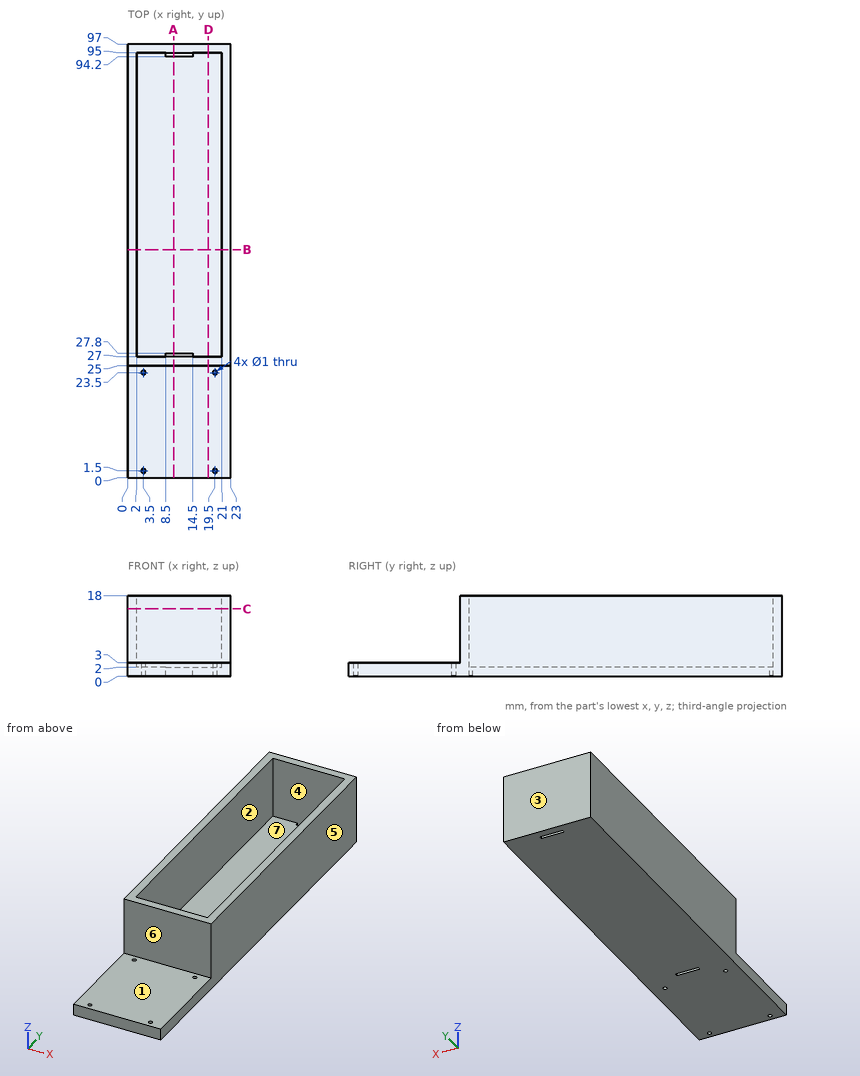
Geometry: see drawing. Coordinates: mm, zero at the bounding-box minimum. A direction names the side the tool comes from. Give positions to 0.01 mm unless a question says otherwise; leave off trailing zeros. Order: outer loops, then holes, each group sorted by start corner. A loop starts at its lowest first (then second) coordinate and runs counter-clockwise, first axis right, second up. Notation, with made-up numbers: M 19.5,55.25 L 28.5,55.25 A31 cw 28.5,84.25 Z; hole C 11.5,44 d3. An arc over 180 degrees is marked long. Answer as CSV lines item,"result". Start each with the question number.
1) Cut plane A-A (x = 10.25). Output: boundary loops of the cut face in (y, z).
2) Line query: line 1 (X direction, y = 1.5, z = 1.55); line 2 (Y direction, x = 19.5, z = 0.65); line 3 (Y direction, x = 7.25, z = 6.75). Output: solid intervals per line, ascending. Write a range as from..to.
3) First-contact query: P1, Ø8, axis at x = 18.5, y = 74.5, coming from the -Z side; P2, Ø10, axis at x = 9, z = 16, coming from the -Y side; P3, Ø11.5, axis at x = 16.5, y = 18, coming from the +Z side. Flat tips, straight axial feed; report the tip coordinate or a pass-through.
4) Cut plane B-B (y = 51). Output: boundary loops of the cut face in (x, z), then the cut area to 3 significant figures.
5) Cut plane D-D (x = 18). Output: boundary loops of the cut face in (y, z), then the cut area to 3 significant figures.
6) Set-up query: the marked faces 5, 6 and 7. Return all of +Z, -Z, +X, -X, +Y, -Y with unobstructed straight access to the full face (end or side cutting, diameter ignored); none if empty.
7) Cut plane C-C (z = 15). Output: boundary loops of the cut face in (x, y), then the cut area to 3 significant figures.
8) Mould query, pull axis Y, two halves, no side actions, for the marked faces 1, 2, 3 and 4. Classes: +Y half, -Y half, draft (parallel to the pull), parting line (faces both ways), or undercut.
Findings below:
1,outline,"M 0,0 L 27,0 L 27,18 L 25,18 L 25,3 L 0,3 Z; M 27.8,0 L 94.2,0 L 94.2,2 L 27.8,2 Z; M 95,0 L 97,0 L 97,18 L 95,18 Z"
2,line 1,"x = 0..3, 4..19, 20..23"
2,line 2,"y = 0..1, 2..23, 24..97"
2,line 3,"y = 25..27, 95..97"
3,P1,"stops at z = 0"
3,P2,"stops at y = 25"
3,P3,"stops at z = 3"
4,outline,"M 0,0 L 23,0 L 23,18 L 21,18 L 21,2 L 2,2 L 2,18 L 0,18 Z"
4,area,"110 mm²"
5,outline,"M 0,0 L 97,0 L 97,18 L 95,18 L 95,2 L 27,2 L 27,18 L 25,18 L 25,3 L 0,3 Z"
5,area,"283 mm²"
6,face 5,"+Z, -Z, +X, +Y, -Y"
6,face 6,"+Z, +X, -X, -Y"
6,face 7,"+Z"
7,outline,"M 0,25 L 23,25 L 23,97 L 0,97 Z; hole M 2,27 L 21,27 L 21,95 L 2,95 Z"
7,area,"364 mm²"
8,face 1,"draft"
8,face 2,"undercut"
8,face 3,"+Y half"
8,face 4,"undercut"
